Check sheet for the modelled part. Datum: model origin and axes. Units: mm. A direction names the side the tool comes from. Round coordinates to 2 decimals unless told otherwise and drop trailing zeros. Loops run counter-clockwise (first coordinate to the right, second up) from the corner with the lowest first, then second, coordinate; pieces in that order, holes last. Notation, with made-up numbers: (-18, -12.5) - (8, -12.5) arc R9 ccw to (8, 3.5) - close; hole circle Ø10 at (-3, -22). An arc over 180 degrees is marked (long way). Put each result on its own line as item: value.
```python
from build123d import *

# Parameters (mm, degrees)
SKETCH_1_R               = 80
EXTRUDE_1_DEPTH          = 130
SKETCH_2_R               = 40
CUT_EXTRUDE_1_DEPTH      = 40
CUT_EXTRUDE_3_DEPTH      = 90
SKETCH_4_R               = 20
CUT_EXTRUDE_4_DEPTH      = 173.336879396
CUT_EXTRUDE_4_DEPTH_BACK = 173.336879396
CUT_EXTRUDE_8_REACH      = 174.337
CUT_EXTRUDE_8_END_RADIUS = 20
EXTRUDE_5_REACH          = 205.777
EXTRUDE_5_END_RADIUS     = 80
SKETCH_8_R               = 20


with BuildPart() as part:
    # 草图1 → 凸台-拉伸1 (new body)
    with BuildSketch(Plane(origin=(0, 0, 0), x_dir=(1, 0, 0), z_dir=(0, 1, 0))):
        with Locations(Location((0, 0, 0), (0, 0, 270))):
            Circle(SKETCH_1_R)
    extrude(amount=EXTRUDE_1_DEPTH)

    # 草图2 → 切除-拉伸1 (cut)
    with BuildSketch(Plane.XZ):
        with Locations(Location((0, 0, 0), (0, 0, 270))):
            Circle(SKETCH_2_R)
    extrude(amount=-CUT_EXTRUDE_1_DEPTH, mode=Mode.SUBTRACT)

    # 草图3 → 切除-拉伸3 (cut)
    with BuildSketch(Plane.XZ.offset(-40)):
        with BuildLine():
            Line((-58.094750193, 55), (26.457513111, 55))
            Line((26.457513111, 55), (26.457513111, 30))
            ThreePointArc((26.457513111, 30), (40, 0), (26.457513111, -30))
            Line((26.457513111, -30), (26.457513111, -55))
            Line((26.457513111, -55), (-58.094750193, -55))
            ThreePointArc((-58.094750193, -55), (-80, 0), (-58.094750193, 55))
        make_face()
    extrude(amount=-CUT_EXTRUDE_3_DEPTH, mode=Mode.SUBTRACT)

    # 草图4 → 切除-拉伸4 (cut, two sides)
    with BuildSketch(Plane.XY) as cut_extrude_4_sk:
        with Locations(Location((0, 95, 0), (0, 0, 180))):
            Circle(SKETCH_4_R)
    extrude(amount=CUT_EXTRUDE_4_DEPTH, mode=Mode.SUBTRACT)
    extrude(cut_extrude_4_sk.sketch, amount=-CUT_EXTRUDE_4_DEPTH_BACK, mode=Mode.SUBTRACT)

    # 切除-拉伸8: up to this cylinder (the profile starts outside it)
    cut_extrude_8_end = Plane(origin=(0, 95, -67.091154), z_dir=(0, 0, -1)) * Cylinder(CUT_EXTRUDE_8_END_RADIUS, 389.674, mode=Mode.PRIVATE)
    # 草图7 → 切除-拉伸8 (cut, up to the surface)
    with BuildSketch(Plane(origin=(0, 130, 0), x_dir=(1, 0, 0), z_dir=(0, 1, 0)), mode=Mode.PRIVATE) as cut_extrude_8_sk1:
        with BuildLine():
            Line((20, 55), (-20, 55))
            Line((-20, 55), (-20, 77.459666924))
            ThreePointArc((-20, 77.459666924), (0, 80), (20, 77.459666924))
            Line((20, 77.459666924), (20, 55))
        make_face()
    cut_extrude_8_tool1 = extrude(cut_extrude_8_sk1.sketch, amount=-CUT_EXTRUDE_8_REACH, mode=Mode.PRIVATE) - cut_extrude_8_end
    add(cut_extrude_8_tool1.solids().sort_by_distance((0, 130, -67.091154))[0], mode=Mode.SUBTRACT)

    # 凸台-拉伸5: up to this cylinder (the profile starts inside it)
    extrude_5_end = Plane(origin=(0, 95, 0), z_dir=(0, -1, 0)) * Cylinder(EXTRUDE_5_END_RADIUS, 572.554, mode=Mode.PRIVATE)
    # 草图8 → 凸台-拉伸5 (add, up to the surface)
    with BuildSketch(Plane.XY.offset(-55), mode=Mode.PRIVATE) as extrude_5_sk1:
        with Locations(Location((0, 95, 0), (0, 0, 270))):
            Circle(SKETCH_8_R)
    extrude_5_tool1 = extrude(extrude_5_sk1.sketch, amount=-EXTRUDE_5_REACH, mode=Mode.PRIVATE) & extrude_5_end
    add(extrude_5_tool1.solids().sort_by_distance((0, 95, -55))[0])


solid = part.part
```
Item 1: Section check A-A on x = 0. Enter the section's corners in (y, z), then the cut area to 4 significant figures.
Filled sheet:
outline: (0, -80) - (115, -80) - (115, -55) - (40, -55) - (40, -40) - (0, -40) - close; (0, 40) - (40, 40) - (40, 55) - (75, 55) - (75, 80) - (0, 80) - close; (115, 55) - (130, 55) - (130, 80) - (115, 80) - close
area: 6,325 mm²
Item 2: Section check B-B on z = 0. Enter the section's corners in (x, y), then the cut area to 3 significant figures.
Filled sheet:
outline: (-80, 0) - (-40, 0) - (-40, 40) - (-80, 40) - close; (40, 0) - (80, 0) - (80, 130) - (40, 130) - close
area: 6,800 mm²
Item 3: Thickness scan on line 1 (X direction, y = 8.5, z = 0); line 2 (Y direction, x = 0, z = 60). Record the ranges inside material, lowest first. Write a range as from..to.
Filled sheet:
line 1: -80..-40, 40..80
line 2: 0..75, 115..130
Item 4: Section check D-D on y = 44. Enter the section's corners in (x, z), then the cut area to 3 significant figures.
Filled sheet:
outline: (-58.09, -55) arc R80 ccw (long way) to (-58.09, 55) - (26.46, 55) - (26.46, 30) arc R40 cw to (26.46, -30) - (26.46, -55) - close
area: 8,590 mm²
Item 5: Section check C-C on x = 36.5. Enter the section's corners in (y, z), then the cut area to 3 significant figures.
Filled sheet:
outline: (0, -71.19) - (130, -71.19) - (130, -16.36) - (0, -16.36) - close; (0, 16.36) - (130, 16.36) - (130, 71.19) - (0, 71.19) - close
area: 14,300 mm²
Item 6: Tool access check on faces 1 (the flat face through (-26, 84, 55)), 2 (the cylindrical face through (2.6, 75.17, 67.32)), 3 (the flat face through (42, 130, 13)). Record the directions out of +Z, -Z, +X, -X, +Y, -Y that give a thin tool (end or side, any length) a straight path to the whole face; none if there is none.
Filled sheet:
face 1: -X, +Y
face 2: +Z
face 3: +Z, -Z, +X, -X, +Y
Item 7: Release check for a two-part mould opening along X. For faces 4 (the flat face through (26.458, 84, 43)), 5 (the flat face through (37, 0, 17)), 6 (the flat face through (-20, 113, -66)), 7 (the cylindrical face through (79.32, 64.09, -10.41)) record: +X half, -X half, draft (parallel to the pull), parting line (faces both ways), or undercut.
Filled sheet:
face 4: -X half
face 5: draft
face 6: undercut
face 7: parting line
Item 8: Go/stop test with flat-tipped pins: pin 1 (10 mm diameter, centred on x = 56.5, z = -60, fed in from -Y); pin 2 (10 mm diameter, centred on x = -37, y = 99.5, fed in from -Z); pin 3 (8 mm diameter, centred on y = 35.5, z = 45, fed in from +X) (3 decimals); pin 4 (12.5 mm diameter, centred on y = 69.5, z = -42, fed in from -X). Record where each tip stops, or that it passes through.
Filled sheet:
pin 1: y = 0
pin 2: z = -73.32
pin 3: x = 68.695
pin 4: x = 26.46
